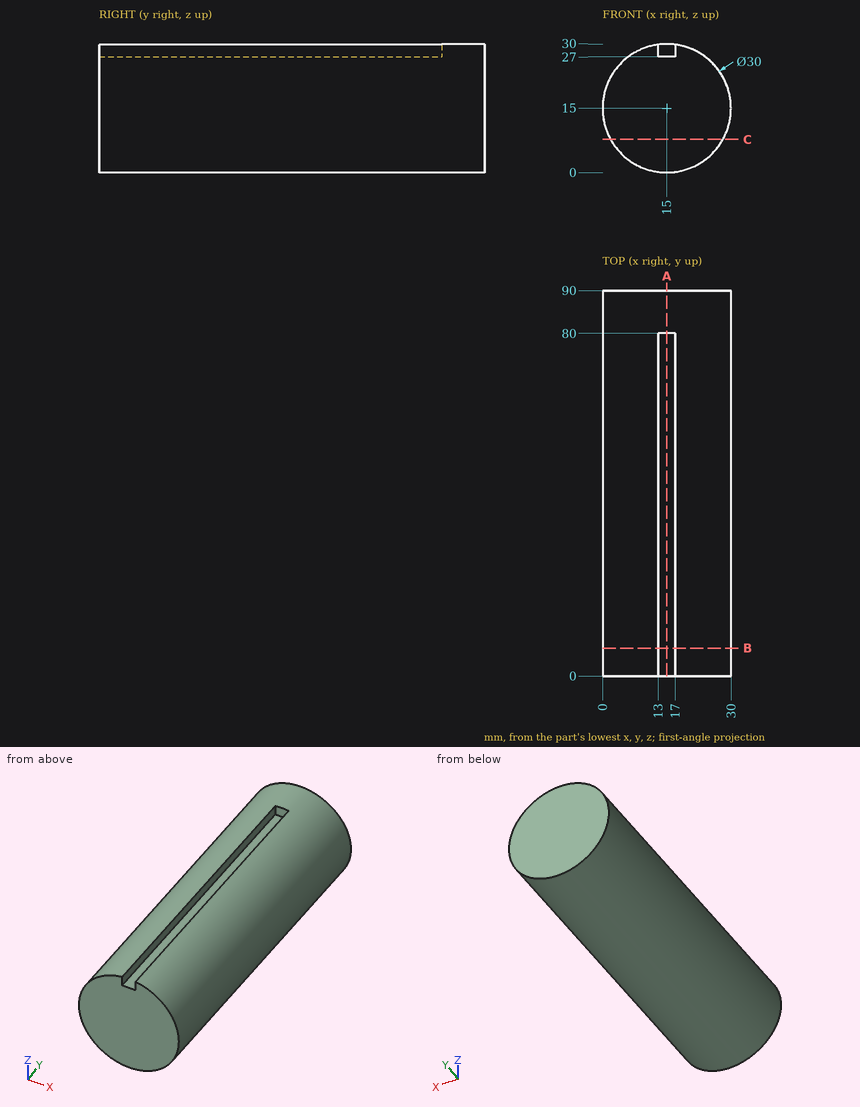
Answer from the drawing. Dimensions are ordinates in mm from the lowest x, y and z of the part. Round coordinates to 2 decimals unless told otherwise and drop trailing zeros. Order: outer loops, then holes, each group sorted by start corner. A loop starts at its lowest first (then second) coordinate and runs counter-clockwise, first axis right, second up.
1) Straight lines are drawn through the part: L1, parallel to Z at x = 15, y = 10; L2, parallel to X at y = 59, z = 27.75; L3, parallel to X at y = 59.5, z = 16. For each, find the intervals that lie inside material, in ascending order.
2) The part is cut by section A-A on x = 15. Write down the section's boundary in (y, z).
3) The part is cut by section B-B on y = 6.5. Write down the section's boundary in (x, z).
4) The part is cut by section C-C on z = 7.75. Write down the section's boundary in (x, y), plus the area to 3 significant figures.
5) Flat-ended cylindrical pins translate along their axes: pin 1 (3 mm diameter, centred on x = 15, y = 31.5, fed in from +Z); pin 2 (3 mm diameter, centred on y = 51.5, z = 29, fed in from -X); pin 3 (1 mm diameter, centred on x = 13, y = 17, fed in from +Z). Find the tip coordinate at first contact, or state that the pin passes through.
Resolved:
1. L1: z = 0 to 27
1. L2: x = 7.1 to 13, 17 to 22.9
1. L3: x = 0.03 to 29.97
2. outline: (0, 0) - (90, 0) - (90, 30) - (80, 30) - (80, 27) - (0, 27) - close
3. outline: (13, 27) - (13, 29.87) arc R15 ccw (long way) to (17, 29.87) - (17, 27) - close
4. outline: (1.87, 0) - (28.13, 0) - (28.13, 90) - (1.87, 90) - close
4. area: 2,360 mm2
5. pin 1: stops at z = 27
5. pin 2: stops at x = 6.71
5. pin 3: stops at z = 29.87
